Autodesk Inventor part; units mm, degrees
ref_plane "YZ Plane" through (0, 0, 0) normal (1, 0, 0) x (0, 1, 0)
ref_plane "XZ Plane" through (0, 0, 0) normal (0, 1, 0) x (-1, 0, 0)
ref_plane "XY Plane" through (0, 0, 0) normal (0, 0, 1) x (1, 0, 0)
sketch "Sketch1" plane through (0, 0, 0) normal (0, 1, 0) x (-1, 0, 0)
  line L0 (-34.9521, -11.6688) -> (41.2479, -11.6688)
  line L1 (41.2479, -11.6688) -> (41.2479, 13.7312)
  line L2 (41.2479, 13.7312) -> (-34.9521, 13.7312)
  line L3 (-34.9521, 13.7312) -> (-34.9521, -11.6688)
  line L4 (-34.9521, -11.6688) -> (41.2479, 13.7312) construction
  line L5 (41.2479, -11.6688) -> (-34.9521, 13.7312) construction
  point P0 (0, 0)
  point P1 (3.1479, 1.0312)
  dimension "d0" = 76.2
  dimension "d2" = 25.4
extrude "Extrusion1" add sketch "Sketch1" along normal blind 3.175
sketch "Sketch2" plane through (0, 3.175, 0) normal (0, 1, 0) x (1, 0, 0)
  line L0 (34.9521, 11.6688) -> (-41.2479, 11.6688)
  line L1 (-41.2479, 11.6688) -> (-41.2479, -13.7312)
  line L2 (34.9521, -13.7312) -> (34.9521, 11.6688)
  point P0 (0, 0)
  point P1 (-28.5479, -1.0312)
  point P2 (22.2521, -1.0312)
  dimension "d5" = 12.7
  dimension "d6" = 12.7
  dimension "d7" = 12.7
  dimension "d8" = 12.7
hole "Hole1" at (-28.5479, 3.175, 1.0312) at (22.2521, 3.175, 1.0312) direction (0, -1, 0) diameter 6.35 end through all
properties part number "Spacer" material "Aluminum 6061"
Source: CAD feature listing. Evaluate the final solid. Frame: model axes, mm. Give positions to 0.01 mm unless a question says otherwise; leave off trailing zeros. Order: outer loops, then holes, each group sorted by start corner. A loop starts at its lowest first (then second) coordinate and runs counter-clockwise, first axis right, second up. Notation, with made-up numbers: (-23, 13) -> (27, 13) arc R26 ccw to (27, 27) -> close; hole circle Ø1 at (40.25, -4). An arc over 180 degrees is marked (long way). Write item = value, one per line.
Q1. Material intervals for line 1 (Z direction, x = 22, y = 0.8); line 2 (X direction, y = 1.6, z = 2); line 3 (Z direction, x = -30.5, y = 1.9), sorted ascending. Write a range as from..to.
Data:
line_1 = -11.67..-2.13, 4.2..13.73
line_2 = -41.25..-31.57, -25.52..19.23, 25.28..34.95
line_3 = -11.67..-1.47, 3.54..13.73
Q2. Cut plane C-C, the plane z = -0.75. Output: boundary loops of the cut face in (x, y) (3 decimals), and give its area (3 significant figures).
Data:
outline = (-41.248, 0) -> (-31.176, 0) -> (-31.176, 3.175) -> (-41.248, 3.175) -> close; (-25.92, 0) -> (19.624, 0) -> (19.624, 3.175) -> (-25.92, 3.175) -> close; (24.88, 0) -> (34.952, 0) -> (34.952, 3.175) -> (24.88, 3.175) -> close
area = 209 mm^2
Q3. Pull-direction query (Z, two-part tool) for faces 1 (the face through (34.952, 2, 1)), 2 (the face through (-31.696, 1.565, 0.618)), 3 (the face through (-4, 2, 13.731)); classes: released by +Z, released by -Z, zero draft, split by the parting line, or undercut.
Data:
face_1 = zero draft
face_2 = undercut
face_3 = released by +Z
Q4. Cut plane B-B, the plane y = 1.15. Output: boundary loops of the cut face in (x, z) (3 decimals).
Data:
outline = (-41.248, -11.669) -> (34.952, -11.669) -> (34.952, 13.731) -> (-41.248, 13.731) -> close; hole circle Ø6.35 at (-28.548, 1.031); hole circle Ø6.35 at (22.252, 1.031)
Q5. Cut plane A-A, the plane x = 21.5. Output: boundary loops of the cut face in (y, z) (3 decimals).
Data:
outline = (0, -11.669) -> (3.175, -11.669) -> (3.175, -2.053) -> (0, -2.053) -> close; (0, 4.116) -> (3.175, 4.116) -> (3.175, 13.731) -> (0, 13.731) -> close
